Build history of the part. All positions in model axes, mm. Give positions to 0.01 mm unless a question says otherwise; leave off trailing zeros. Loops run counter-clockwise (first coordinate to the right, second up) from the corner with the lowest first, then second, coordinate; pieces in that order, holes last. Notation, with made-up numbers: (-11.5, -9.5) - (45.5, -9.5) arc R14 ccw to (45.5, 8.5) - close; hole circle Ø2 at (79, -36). An arc over 180 degrees is marked (long way). Return JSON: item names as keys, results as strings. Group by question number.
1) Slice it at B-B (x = 22.5). List the corners of the cut face in (y, z).
2) Slice it at C-C (y = 15.75). List the corners of the cut face in (x, z).
3) Drop flat-ended pins along their axis: pin 1 (6.5 mm diameter, centred on x = -22.5, z = -26, fed in from -Y); pin 2 (1 mm diameter, centred on x = 4.5, y = 0.5, fed in from +Z); pin 3 (2 mm diameter, centred on y = 6, z = 201.5, fed in from +X); pin 4 (12 mm diameter, centred on y = 5.5, z = 158.5, fed in from -X). Give the stop position or say it passes through.
4) Drill centre lines: probe 1 along X at (y, z) = (0.7, 26); probe 2 along Y at (x, z) = (-3, 271); probe 3 along X at (y, z) = (7.25, 11). Where is each one in solid material? Low to high. Write a range as from..to.
5) Slice it at D-D (x = -13). List the corners of the cut face in (y, z), and give its area (3 significant figures).
6) Slice it at A-A (z = 26). List the corners of the cut face in (x, y).
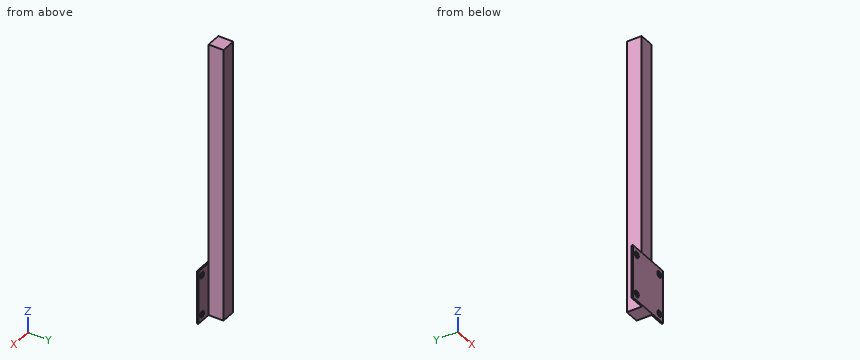
```python
from build123d import *

# Parameters (mm, degrees)
SKETCH1_W                = 60.5
SKETCH1_H                = 69.5
SKETCH1_R                = 4
BOSS_EXTRUDE1_DEPTH      = 2
SKETCH2_W                = 19.5
SKETCH2_H                = 19.5
BOSS_EXTRUDE2_DEPTH      = 325.596
BOSS_EXTRUDE2_DEPTH_BACK = 34.75


with BuildPart() as part:
    # Sketch1 → Boss-Extrude1 (new body)
    with BuildSketch(Plane(origin=(0, 0, 0), x_dir=(1, 0, 0), z_dir=(0, 1, 0))):
        Rectangle(SKETCH1_W, SKETCH1_H)
        with Locations((-22.5, 26)):
            Circle(SKETCH1_R, mode=Mode.SUBTRACT)
        with Locations((22.5, 26)):
            Circle(SKETCH1_R, mode=Mode.SUBTRACT)
        with Locations((-22.5, -26)):
            Circle(SKETCH1_R, mode=Mode.SUBTRACT)
        with Locations((22.5, -26)):
            Circle(SKETCH1_R, mode=Mode.SUBTRACT)
    extrude(amount=BOSS_EXTRUDE1_DEPTH)

    # Sketch2 → Boss-Extrude2 (add, two sides)
    with BuildSketch(Plane.XY) as boss_extrude2_sk:
        with Locations((0, 11.75)):
            Rectangle(SKETCH2_W, SKETCH2_H)
    extrude(amount=BOSS_EXTRUDE2_DEPTH)
    extrude(boss_extrude2_sk.sketch, amount=-BOSS_EXTRUDE2_DEPTH_BACK)


solid = part.part
```
Results:
{
 "1": {"outline": "(0, -34.75) - (2, -34.75) - (2, -30) - (0, -30) - close; (0, -22) - (2, -22) - (2, 22) - (0, 22) - close; (0, 30) - (2, 30) - (2, 34.75) - (0, 34.75) - close"},
 "2": {"outline": "(-9.75, -34.75) - (9.75, -34.75) - (9.75, 325.6) - (-9.75, 325.6) - close"},
 "3": {"pin 1": "through", "pin 2": "z = 34.75", "pin 3": "x = 9.75", "pin 4": "x = -9.75"},
 "4": {"probe 1": "-30.25..-26.5, -18.5..18.5, 26.5..30.25", "probe 2": "2..21.5", "probe 3": "-9.75..9.75"},
 "5": {"outline": "(0, -34.75) - (2, -34.75) - (2, 34.75) - (0, 34.75) - close", "area": "139 mm2"},
 "6": {"outline": "(-30.25, 0) - (-26.5, 0) - (-26.5, 2) - (-30.25, 2) - close; (-18.5, 0) - (18.5, 0) - (18.5, 2) - (9.75, 2) - (9.75, 21.5) - (-9.75, 21.5) - (-9.75, 2) - (-18.5, 2) - close; (26.5, 0) - (30.25, 0) - (30.25, 2) - (26.5, 2) - close"}
}
